```python
from build123d import *

# Parameters (mm, degrees)
SKETCH1_W           = 16
SKETCH1_H           = 38
BOSS_EXTRUDE1_DEPTH = 8
SKETCH2_W           = 5.5
SKETCH2_H           = 22
BOSS_EXTRUDE2_DEPTH = 4.5
SKETCH6_R           = 2.25
BOSS_EXTRUDE3_DEPTH = 20
FILLET6_R           = 2
CHAMFER1_SIZE       = 2
SKETCH7_R           = 2.85
CUT_EXTRUDE1_DEPTH  = 10
SKETCH8_R           = 6
CUT_EXTRUDE2_DEPTH  = 3
CUT_EXTRUDE3_START  = -10
SKETCH9_R           = 12.5
CUT_EXTRUDE3_DEPTH  = 4
FILLET7_R           = 2


with BuildPart() as part:
    # Sketch1 → Boss-Extrude1 (new body)
    with BuildSketch(Plane(origin=(0, 0, 0), x_dir=(0, 0, -1), z_dir=(1, 0, 0))):
        with Locations((-40.846556001, 16.91146402)):
            Rectangle(SKETCH1_W, SKETCH1_H)
    extrude(amount=BOSS_EXTRUDE1_DEPTH)

    # Sketch2 → Boss-Extrude2 (add)
    with BuildSketch(Plane.ZY):
        with Locations((40.846556001, 24.91146402)):
            Rectangle(SKETCH2_W, SKETCH2_H)
    extrude(amount=BOSS_EXTRUDE2_DEPTH)

    # Sketch6 → Boss-Extrude3 (add)
    with BuildSketch(Plane.XZ.offset(-35.91146402)):
        with BuildLine():
            Line((8, 48.846556001), (16, 48.846556001))
            ThreePointArc((16, 48.846556001), (24, 40.846556001), (16, 32.846556001))
            Line((16, 32.846556001), (8, 32.846556001))
            Line((8, 32.846556001), (8, 48.846556001))
        make_face()
        with Locations(Location((16, 40.846556001, 0), (0, 0, 270))):
            Circle(SKETCH6_R, mode=Mode.SUBTRACT)
    extrude(amount=BOSS_EXTRUDE3_DEPTH)

    # Fillet6
    fillet6_edges = [part.edges().sort_by_distance(p)[0] for p in [
        (8, 15.91146402, 40.846556001),
    ]]
    fillet(fillet6_edges, radius=FILLET6_R)

    # Chamfer1
    chamfer1_edges = [part.edges().sort_by_distance(p)[0] for p in [
        (-4.5, 13.91146402, 40.846556001),
        (-4.5, 35.91146402, 40.846556001),
    ]]
    chamfer(chamfer1_edges, length=CHAMFER1_SIZE)

    # Sketch7 → Cut-Extrude1 (cut)
    with BuildSketch(Plane(origin=(8, 0, 0), x_dir=(0, 0, -1), z_dir=(1, 0, 0))):
        with Locations((-40.846556001, 5.91146402)):
            Circle(SKETCH7_R)
    extrude(amount=-CUT_EXTRUDE1_DEPTH, mode=Mode.SUBTRACT)

    # Sketch8 → Cut-Extrude2 (cut)
    with BuildSketch(Plane(origin=(8, 0, 0), x_dir=(0, 0, -1), z_dir=(1, 0, 0))):
        with Locations((-40.846556001, 5.91146402)):
            Circle(SKETCH8_R)
    extrude(amount=-CUT_EXTRUDE2_DEPTH, mode=Mode.SUBTRACT)

    # Sketch9 → Cut-Extrude3 (cut, symmetric)
    with BuildSketch(Plane(origin=(0, 35.91146402, 0), x_dir=(1, 0, 0), z_dir=(0, 1, 0)).offset(CUT_EXTRUDE3_START)):
        with Locations((16, -40.846556001)):
            Circle(SKETCH9_R)
    extrude(amount=CUT_EXTRUDE3_DEPTH, both=True, mode=Mode.SUBTRACT)

    # Fillet7
    fillet7_edges = [part.edges().sort_by_distance(p)[0] for p in [
        (4, -2.08853598, 32.846556001),
        (4, -2.08853598, 48.846556001),
    ]]
    fillet(fillet7_edges, radius=FILLET7_R)


solid = part.part
```
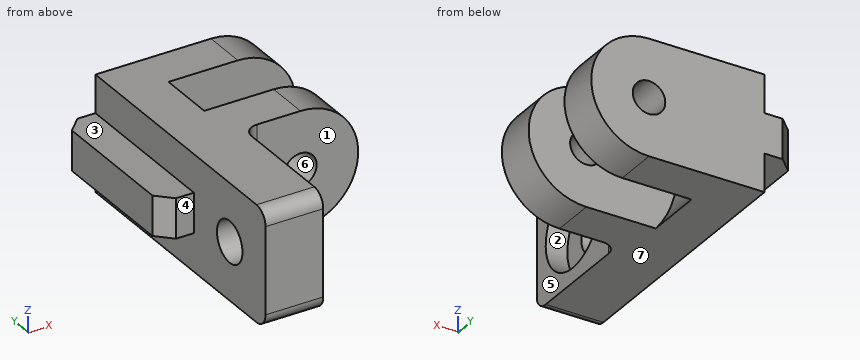
Input: part model. Units: mm. Frame: model coordinates. Face numbers are marked on the shaded views. A direction names the side the tool comes from. Round coordinates to 2 decimals unless told otherwise and drop trailing zeros. Write each loop counter-clockwise with the first axis right and the second up, starting at its lowest first coordinate (ties: lowest second). Pieces come first, ordered by that corner, then holes. Notation, with made-up numbers: M 19.5,7 L 55.5,7 A16 ccw 55.5,25 Z; hole C 55.5,-35 d1. An arc over 180 degrees is marked long. Write each question's results on one line, items separated by ' | '.
Q1. Section query D-D (y = 28). Return loops of the section in (x, z), and give its area (3 significant figures).
Results:
outline: M -4.5,38.1 L 0,38.1 L 0,32.85 L 6.4,32.85 A12.5 cw 6.4,48.85 L 0,48.85 L 0,43.6 L -4.5,43.6 Z | area: 95.4 mm^2
Q2. Section query C-C (x = 0.5). Return loops of the section in (y, z), and give its area (3 significant figures).
Results:
outline: M -2.09,34.85 A2 ccw -0.09,32.85 L 35.91,32.85 L 35.91,48.85 L -0.09,48.85 A2 ccw -2.09,46.85 Z; hole C 5.91,40.85 d5.7 | area: 581 mm^2
Q3. Pin query (flat end, axial travel): P1, Ø1.2, axis at x = -1.5, z = 42, coming from the -Y side; P2, Ø7, axis at y = 5.91, z = 40.85, coming from the -X side; P3, Ø1.3, axis at x = -1.5, y = 22.5, coming from the -Z side; P4, Ø8, axis at x = 8.5, z = 37, coming from the -Y side. Return the tip coordinate at first contact, or that it passes through.
Results:
P1: stops at y = 13.91 | P2: stops at x = 0 | P3: stops at z = 38.1 | P4: stops at y = -2.09
Q4. Section query B-B (z = 41.25). State how many separate pieces and enclosed holes the cut face has, and give its area (3 significant figures).
Results:
separate pieces: 4 | enclosed holes: 0 | area: 439 mm^2
Q5. Draft query along Z for the marked faces 5, 6 and 7. Return one class per face: released by +Z, released by -Z, zero draft, split by the parting line, or undercut.
Results:
face 5: zero draft | face 6: undercut | face 7: released by -Z
Q6. Line query: line 1 along Y through (x, z) = (13, 45.5); line 2 along Z through (x, y) = (16, 33.3); line 3 along Y through (x, z) = (8.75, 34). Output: solid intervals per line, ascending.
Results:
line 1: y = 15.91 to 21.91, 29.91 to 35.91 | line 2: z = 32.85 to 38.6, 43.1 to 48.85 | line 3: y = 15.47 to 21.91, 29.91 to 35.91
Q7. Access query for the marked faces 1, 2, 3 and 4. Directions: +Z, -Z, +X, -X, +Y, -Y. A direction counts if a zero-diameter tool reaches every point of the face in a straight line with its end or side. Return the directions, or none.
Results:
face 1: +Z, -Z, +X, -Y | face 2: +X | face 3: +Z, -X, +Y, -Y | face 4: +Z, -Z, -X, -Y
Q8. Section query A-A (y = 4). Return loops of the section in (x, z), and give its area (3 significant figures).
Results:
outline: M 0,32.85 L 8,32.85 L 8,35.16 L 5,35.16 L 5,38.73 L 0,38.73 Z; M 0,42.96 L 5,42.96 L 5,46.53 L 8,46.53 L 8,48.85 L 0,48.85 Z | area: 72.7 mm^2
